Part model, mm, in its own coordinate system. A direction names the side the tool comes from. Give positions to 0.01 mm unless a question says otherwise; leave off trailing zeros. Order: outer loops, then holes, each group sorted by start corner. A loop starts at its lowest first (then second) coordinate and runs counter-clockwise, first axis right, second up. Notation, with made-up numbers: (-15, 12.25) - (20, 12.25) arc R16 ccw to (20, 26.25) - close; hole circle Ø10 at (-3.75, 48.25). An arc over 180 degrees is marked (long way). One line per item, written item: value.
```python
from build123d import *

# Parameters (mm, degrees)
SKETCH3_W           = 10
SKETCH3_H           = 12
SKETCH3_R           = 1.5
BOSS_EXTRUDE2_DEPTH = 1.5
SKETCH3_5_W         = 20
SKETCH3_5_H         = 1.5
BOSS_EXTRUDE4_DEPTH = 4
SKETCH3_6_W         = 10
SKETCH3_6_H         = 4
BOSS_EXTRUDE5_DEPTH = 0.25
BOSS_EXTRUDE7_DEPTH = 2.5


with BuildPart() as part:
    # Sketch3 → Boss-Extrude2 (new body)
    # profile 1 of 2: a face of its own
    with BuildSketch(Plane(origin=(0, 0, 0), x_dir=(1, 0, 0), z_dir=(0, 1, 0))):
        with Locations((7, 11.5)):
            Rectangle(SKETCH3_W, SKETCH3_H)
        with Locations(Location((4.5, 15, 0), (0, 0, 270))):
            Circle(SKETCH3_R, mode=Mode.SUBTRACT)
    # profile 2 of 2: a face of its own
    with BuildSketch(Plane(origin=(0, 0, 0), x_dir=(1, 0, 0), z_dir=(0, 1, 0))):
        with Locations((17, 11.5)):
            Rectangle(SKETCH3_W, SKETCH3_H)
        with Locations(Location((19.5, 15, 0), (0, 0, 270))):
            Circle(SKETCH3_R, mode=Mode.SUBTRACT)
    extrude(amount=BOSS_EXTRUDE2_DEPTH)

    # Sketch3_6 → Boss-Extrude5 (add)
    with BuildSketch(Plane(origin=(0, 0, 0), x_dir=(1, 0, 0), z_dir=(0, 1, 0))):
        with Locations((17, 3.5)):
            Rectangle(SKETCH3_6_W, SKETCH3_6_H)
        with Locations((7, 3.5)):
            Rectangle(SKETCH3_6_W, SKETCH3_6_H)
    extrude(amount=BOSS_EXTRUDE5_DEPTH)



with BuildPart() as body_2:
    # Sketch3_5 → Boss-Extrude4 (new body)
    with BuildSketch(Plane(origin=(0, 0, 0), x_dir=(1, 0, 0), z_dir=(0, 1, 0))):
        with Locations((12, 0.75)):
            Rectangle(SKETCH3_5_W, SKETCH3_5_H)
    extrude(amount=BOSS_EXTRUDE4_DEPTH)


with BuildPart() as part_1:
    add(part.part)

    add(body_2.part)  # Boss-Extrude7 merges body 2
    # Sketch3_8 → Boss-Extrude7 (add)
    with BuildSketch(Plane(origin=(0, 0, 0), x_dir=(1, 0, 0), z_dir=(0, 1, 0))):
        with BuildLine():
            ThreePointArc((0, 1), (0.292893219, 0.292893219), (1, 0))
            Line((1, 0), (2, 0))
            Line((2, 0), (2, 1.5))
            Line((2, 1.5), (2, 5.5))
            Line((2, 5.5), (2, 17.5))
            Line((2, 17.5), (22, 17.5))
            Line((22, 17.5), (22, 5.5))
            Line((22, 5.5), (22, 1.5))
            Line((22, 1.5), (22, 0))
            Line((22, 0), (23, 0))
            ThreePointArc((23, 0), (23.707106781, 0.292893219), (24, 1))
            Line((24, 1), (24, 18.5))
            ThreePointArc((24, 18.5), (23.707106781, 19.207106781), (23, 19.5))
            Line((23, 19.5), (1, 19.5))
            ThreePointArc((1, 19.5), (0.292893219, 19.207106781), (0, 18.5))
            Line((0, 18.5), (0, 1))
        make_face()
    extrude(amount=BOSS_EXTRUDE7_DEPTH)


solid = part_1.part
```
1) Slice it at A-A on z = -15. Write the cut outline in (x, y).
Answer:
outline: (0, 0) - (3, 0) - (3, 1.5) - (2, 1.5) - (2, 2.5) - (0, 2.5) - close; (6, 0) - (18, 0) - (18, 1.5) - (6, 1.5) - close; (21, 0) - (24, 0) - (24, 2.5) - (22, 2.5) - (22, 1.5) - (21, 1.5) - close
2) Two-plate mould, pull along Z, no slides. Class faces 5 (the face through (12, 1.5, -12)), 6 (the face through (12, 0, -10)), 7 (the face through (12, 1, -5.5)), 8 (the face through (12, 2, 0)): pulls with the +Z half, pulls with the -Z half, needs draft (parallel to the pull), parting line crosses it, or undercut.
Answer:
face 5: undercut
face 6: needs draft
face 7: undercut
face 8: pulls with the +Z half
3) Slice it at D-D on y = 0.8. Write the cut outline in (x, z).
Answer:
outline: (0, -18.5) arc R1 ccw to (1, -19.5) - (23, -19.5) arc R1 ccw to (24, -18.5) - (24, -1) arc R1 ccw to (23, 0) - (1, 0) arc R1 ccw to (0, -1) - close; hole (2, -5.5) - (22, -5.5) - (22, -1.5) - (2, -1.5) - close; hole circle Ø3 at (4.5, -15); hole circle Ø3 at (19.5, -15)
4) Slice it at C-C on y = 1.9. Write the cut outline in (x, z), then the cut area to 3 significant figures.
Answer:
outline: (0, -18.5) arc R1 ccw to (1, -19.5) - (23, -19.5) arc R1 ccw to (24, -18.5) - (24, -1) arc R1 ccw to (23, 0) - (1, 0) arc R1 ccw to (0, -1) - close; hole (2, -17.5) - (22, -17.5) - (22, -1.5) - (2, -1.5) - close
area: 147 mm2
5) Drop flat-ended pins along their axis: P1, Ø3, axis at x = 5, z = -15.5, coming from the +Y side; P2, Ø1.6, axis at y = 3.5, z = -0.5, coming from the +X side. Give the stop position or say it passes through.
Answer:
P1: stops at y = 1.5
P2: stops at x = 22
6) Slice it at B-B on x = 19.5. Write the cut outline in (y, z), then the cut area to 3 significant figures.
Answer:
outline: (0, -19.5) - (2.5, -19.5) - (2.5, -17.5) - (1.5, -17.5) - (1.5, -16.5) - (0, -16.5) - close; (0, -13.5) - (1.5, -13.5) - (1.5, -5.5) - (0.25, -5.5) - (0.25, -1.5) - (4, -1.5) - (4, 0) - (0, 0) - close
area: 25.5 mm2
7) Wall check: line 1 along X through (y, z) = (0.95, -15); line 2 along Z through (x, y) = (15.25, 1.8); line 3 along X through (y, z) = (0.6, -3.75). Give the ranges that are in metal, low to high. Write a range as [from, to].
Answer:
line 1: x = [0, 3], [6, 18], [21, 24]
line 2: z = [-19.5, -17.5], [-1.5, 0]
line 3: x = [0, 2], [22, 24]
8) Which spindle directions (+Z, -Z, +X, -X, +Y, -Y) get a long thin tool onto all of the face, cutting with end or side? Do faces 1 (the face through (22, 3, -1)), 2 (the face through (12, 2, -17.5)), 3 (the face through (23.699, 1.232, -0.285)), 4 (the face through (2, 3, -1)). Say none if no direction does.
Answer:
face 1: +Z, -Z, +X, +Y
face 2: +Y
face 3: +Z, +X, +Y, -Y
face 4: +Z, -Z, -X, +Y
